from build123d import *

# Parameters (mm, degrees)
BOSS_EXTRUDE1_DEPTH            = 59
BOSS_EXTRUDE1_DEPTH_BACK       = 4
SKETCH2_R                      = 13.45
FILLET1_R                      = 15
FILLET2_R                      = 3
CUT_EXTRUDE1_REACH             = 88.686
CUT_EXTRUDE1_DIRECTION_2_DEPTH = 87.685720739
SKETCH4_R                      = 1.4
CUT_EXTRUDE2_DEPTH             = 9


with BuildPart() as part:
    # Sketch2 → Boss-Extrude1 (new, two sides: drawn at the far end of the back side and taken through both)
    with BuildSketch(Plane(origin=(0, 0, 0), x_dir=(1, 0, 0), z_dir=(0, 1, 0)).offset(-BOSS_EXTRUDE1_DEPTH_BACK)):
        with BuildLine():
            Line((-17.4, -17.4), (17.4, -17.4))
            Line((17.4, -17.4), (31.4, -17.4))
            ThreePointArc((31.4, -17.4), (38.471067812, -14.471067812), (41.4, -7.4))
            Line((41.4, -7.4), (41.4, 38.781202895))
            Line((41.4, 38.781202895), (41.615303514, 42.605074323))
            Line((41.615303514, 42.605074323), (-17.4, 17.4))
            Line((-17.4, 17.4), (-17.4, -17.4))
        make_face()
        with Locations(Location((0, 0, 0), (0, 0, 270))):
            Circle(SKETCH2_R, mode=Mode.SUBTRACT)
        with BuildLine():
            Line((17.4, -13.4), (17.4, 11.200201908))
            ThreePointArc((17.4, 11.200201908), (17.624507156, 12.521433828), (18.272826893, 13.694352737))
            Line((18.272826893, 13.694352737), (33.836413447, 33.208019968))
            ThreePointArc((33.836413447, 33.208019968), (36.06061596, 33.848690975), (37.4, 31.960944553))
            Line((37.4, 31.960944553), (37.4, -3.4))
            ThreePointArc((37.4, -3.4), (34.471067812, -10.471067812), (27.4, -13.4))
            Line((27.4, -13.4), (17.4, -13.4))
        make_face(mode=Mode.SUBTRACT)
    extrude(amount=BOSS_EXTRUDE1_DEPTH + BOSS_EXTRUDE1_DEPTH_BACK)

    # Fillet1
    fillet1_edges = [part.edges().sort_by_distance(p)[0] for p in [
        (-17.4, 27.5, 17.4),
    ]]
    fillet(fillet1_edges, radius=FILLET1_R)

    # Fillet2
    fillet2_edges = [part.edges().sort_by_distance(p)[0] for p in [
        (-17.4, 27.5, -17.4),
    ]]
    fillet(fillet2_edges, radius=FILLET2_R)

    # Cut-Extrude1: up to this plane
    cut_extrude1_end = Plane(origin=(18.272826893, -4, -13.694352737), z_dir=(-0.7817932766673829, 0, -0.6235377074064384))
    # Sketch3 → Cut-Extrude1 (cut, up to the surface)
    with BuildSketch(Plane(origin=(-8.969274917, 0, -21.000710996), x_dir=(-0.9196362986724037, 0, 0.39277102510765927), z_dir=(-0.39277102510765927, 0, -0.9196362986724037)), mode=Mode.PRIVATE) as cut_extrude1_sk1:
        Polygon((-47.774830044, 0), (-9.235134773, 0), (-28.504982408, 23.552035999), align=None)
    cut_extrude1_tool1 = split(extrude(cut_extrude1_sk1.sketch, amount=-CUT_EXTRUDE1_REACH, mode=Mode.PRIVATE), bisect_by=cut_extrude1_end, keep=Keep.BOTH, mode=Mode.PRIVATE)
    add(cut_extrude1_tool1.solids().sort_by_distance((17.244942, 7.850679, -32.196642))[0], mode=Mode.SUBTRACT)
    # Sketch3 → Cut-Extrude1 (cut, up to the surface)
    with BuildSketch(Plane(origin=(-8.969274917, 0, -21.000710996), x_dir=(-0.9196362986724037, 0, 0.39277102510765927), z_dir=(-0.39277102510765927, 0, -0.9196362986724037)), mode=Mode.PRIVATE) as cut_extrude1_sk2:
        Polygon((-51.004982408, 3.947964001), (-51.004982408, 51.052035999), (-31.735134773, 27.5), align=None)
    cut_extrude1_tool2 = split(extrude(cut_extrude1_sk2.sketch, amount=-CUT_EXTRUDE1_REACH, mode=Mode.PRIVATE), bisect_by=cut_extrude1_end, keep=Keep.BOTH, mode=Mode.PRIVATE)
    add(cut_extrude1_tool2.solids().sort_by_distance((32.029675, 27.5, -38.511111))[0], mode=Mode.SUBTRACT)
    # Sketch3 → Cut-Extrude1 (cut, up to the surface)
    with BuildSketch(Plane(origin=(-8.969274917, 0, -21.000710996), x_dir=(-0.9196362986724037, 0, 0.39277102510765927), z_dir=(-0.39277102510765927, 0, -0.9196362986724037)), mode=Mode.PRIVATE) as cut_extrude1_sk3:
        Polygon((-47.774830044, 55), (-9.235134773, 55), (-28.504982408, 31.447964001), align=None)
    cut_extrude1_tool3 = split(extrude(cut_extrude1_sk3.sketch, amount=-CUT_EXTRUDE1_REACH, mode=Mode.PRIVATE), bisect_by=cut_extrude1_end, keep=Keep.BOTH, mode=Mode.PRIVATE)
    add(cut_extrude1_tool3.solids().sort_by_distance((17.244942, 47.149321, -32.196642))[0], mode=Mode.SUBTRACT)
    # Sketch3 → Cut-Extrude1 (cut, up to the surface)
    with BuildSketch(Plane(origin=(-8.969274917, 0, -21.000710996), x_dir=(-0.9196362986724037, 0, 0.39277102510765927), z_dir=(-0.39277102510765927, 0, -0.9196362986724037)), mode=Mode.PRIVATE) as cut_extrude1_sk4:
        Polygon((-6.004982408, 3.947964001), (-6.004982408, 51.052035999), (-25.274830044, 27.5), align=None)
    cut_extrude1_tool4 = split(extrude(cut_extrude1_sk4.sketch, amount=-CUT_EXTRUDE1_REACH, mode=Mode.PRIVATE), bisect_by=cut_extrude1_end, keep=Keep.BOTH, mode=Mode.PRIVATE)
    add(cut_extrude1_tool4.solids().sort_by_distance((2.460209, 27.5, -25.882173))[0], mode=Mode.SUBTRACT)

    # Sketch3 → Cut-Extrude1 direction 2 (cut)
    with BuildSketch(Plane(origin=(-8.969274917, 0, -21.000710996), x_dir=(-0.9196362986724037, 0, 0.39277102510765927), z_dir=(-0.39277102510765927, 0, -0.9196362986724037))):
        Polygon((-47.774830044, 0), (-9.235134773, 0), (-28.504982408, 23.552035999), align=None)
        Polygon((-51.004982408, 3.947964001), (-51.004982408, 51.052035999), (-31.735134773, 27.5), align=None)
        Polygon((-47.774830044, 55), (-9.235134773, 55), (-28.504982408, 31.447964001), align=None)
        Polygon((-6.004982408, 3.947964001), (-6.004982408, 51.052035999), (-25.274830044, 27.5), align=None)
    extrude(amount=CUT_EXTRUDE1_DIRECTION_2_DEPTH, mode=Mode.SUBTRACT)

    # Sketch4 → Cut-Extrude2 (cut)
    with BuildSketch(Plane(origin=(-8.969274917, 0, -21.000710996), x_dir=(-0.9196362986724037, 0, 0.3927710251076594), z_dir=(-0.3927710251076594, 0, -0.9196362986724037))):
        with Locations((-49.389906226, 1.973982)):
            Circle(SKETCH4_R)
        with Locations((-7.620058591, 1.973982)):
            Circle(SKETCH4_R)
        with Locations((-7.620058591, 53.026018)):
            Circle(SKETCH4_R)
        with Locations((-49.389906226, 53.026018)):
            Circle(SKETCH4_R)
    extrude(amount=-CUT_EXTRUDE2_DEPTH, mode=Mode.SUBTRACT)


solid = part.part
Model file for the job. Use its own axes, mm. A direction names the side the tool comes from. Give positions to 0.01 mm unless a question says otherwise; leave off trailing zeros. Order: outer loops, then holes, each group sorted by start corner. A loop starts at its lowest first (then second) coordinate and runs counter-clockwise, first axis right, second up. Notation, with made-up numbers: (40, 54) - (60, 54) arc R26 ccw to (60, 92) - close; hole circle Ø4 at (56, 17). An arc over 180 degrees is marked (long way). Write item = value, one per line. Start each with the question number.
1. Probe line 1 along X through (y, z) = (10, 0); line 2 along Y through (x, z) = (9.5, -12.5); line 3 along X through (y, z) = (33, -22.5). List the from-to ranges inside material, lowest first.
2. Drop flat-ended pins along their axis: P1, Ø14, axis at y = 32.5, z = -4, coming from the +X side; P2, Ø12, axis at x = -2, z = 6, coming from the -Y side; P3, Ø8, axis at x = 22.5, y = 29, coming from the -Z side; P4, Ø1.5, axis at x = -4, y = 30, coming from the -Z side. Give the stop position or say it passes through.
3. Cut at D-D, the plane y = 45.5. List the corners of the cut face in (x, z), and give its area (3 significant figures).
4. Cut at B-B, the plane y = 33. List the corners of the cut face in (x, z).
5. Which spindle directions (+Z, -Z, +X, -X, +Y, -Y) get a long thin tool onto all of the face, cutting with end or side? Do faces 1 (the flat face through (41.4, 27, -15)), 2 (the flat face through (15.82, 6.04, -10.62)), 3 (the cylindrical face through (34.55, 27.06, 10.39)), 4 (the flat face through (1.591, 1.994, -15.725)). Say none if no direction does.
6. Cut at A-A, the plane z = 0. List the corners of the cut face in (x, y).
7. Two-plate mould, pull along Y, no slides. Class faces 5 (the flat face through (12, -4, -13)), 6 (the flat face through (13.419, 34.059, -30.563)), 7 (the flat face through (29.07, 36.82, -32.15)): pulls with the +Y half, pulls with the -Y half, needs draft (parallel to the pull), parting line crosses it, or undercut.
8. Cut at C-C, the plane z = -29. List the corners of the cut face in (x, y).
Taken from the geometry:
q1.line_1 = -17.4 to -13.45, 13.45 to 17.4, 37.4 to 41.4
q1.line_2 = -4 to 0, 5.39 to 13.29, 41.71 to 49.61, 55 to 59
q1.line_3 = -5.46 to -3.08, 12.98 to 20.01, 22.77 to 25.3, 37.4 to 41.4
q2.P1 = 41.4
q2.P2 = through
q2.P3 = -35.13
q2.P4 = -23.36
q3.outline = (-17.4, -15.42) arc R3 ccw to (-15.58, -18.18) - (-3.45, -23.36) - (0.8, -13.43) arc R13.45 cw (long way) to (6.42, -11.82) - (0.73, -25.14) - (6.67, -27.68) - (14.61, -9.1) - (18.27, -13.69) arc R4 cw to (17.4, -11.2) - (17.4, 13.4) - (27.4, 13.4) arc R10 cw to (37.4, 3.4) - (37.4, -31.96) arc R2 cw to (33.84, -33.21) - (30.89, -29.52) - (27.82, -36.71) - (33.76, -39.25) - (35.47, -35.25) - (38.68, -39.29) - (37.94, -41.03) - (41.62, -42.61) - (41.4, -38.78) - (41.4, 7.4) arc R10 ccw to (31.4, 17.4) - (-2.4, 17.4) arc R15 ccw to (-17.4, 2.4) - close
q3.area = 1,010 mm²
q4.outline = (-17.4, -15.42) arc R3 ccw to (-15.58, -18.18) - (-3.45, -23.36) - (0.8, -13.43) arc R13.45 cw (long way) to (12.08, -5.92) - (17.28, -12.44) - (10.14, -29.16) - (16.08, -31.7) - (21.85, -18.18) - (18.27, -13.69) arc R4 cw to (17.4, -11.2) - (17.4, 13.4) - (27.4, 13.4) arc R10 cw to (37.4, 3.4) - (37.4, -31.96) arc R2 cw to (33.84, -33.21) - (38.68, -39.29) - (37.94, -41.03) - (41.62, -42.61) - (41.4, -38.78) - (41.4, 7.4) arc R10 ccw to (31.4, 17.4) - (-2.4, 17.4) arc R15 ccw to (-17.4, 2.4) - close; (18.41, -32.7) - (24.35, -35.23) - (28.22, -26.17) - (23.65, -20.44) - close
q5.face_1 = +Z, +X, +Y, -Y
q5.face_2 = -Z
q5.face_3 = +Y, -Y
q5.face_4 = none
q6.outline = (-17.4, -4) - (-13.45, -4) - (-13.45, 59) - (-17.4, 59) - close; (13.45, -4) - (17.4, -4) - (17.4, 59) - (13.45, 59) - close; (37.4, -4) - (41.4, -4) - (41.4, 59) - (37.4, 59) - close
q7.face_5 = pulls with the -Y half
q7.face_6 = needs draft
q7.face_7 = undercut
q8.outline = (9.76, -4) - (30.48, -4) - (30.48, 0) - (9.76, 0) - close; (9.76, 13.6) - (18.61, 23.55) - (30.48, 10.21) - (30.48, 18.11) - (22.12, 27.5) - (30.48, 36.89) - (30.48, 44.79) - (18.61, 31.45) - (9.76, 41.4) - (9.76, 33.5) - (15.1, 27.5) - (9.76, 21.5) - close; (9.76, 55) - (30.48, 55) - (30.48, 59) - (9.76, 59) - close; (37.4, -4) - (41.4, -4) - (41.4, 59) - (37.4, 59) - close
